Could you check a few things on this model? Use its own coordinates, in mm. Give positions to 0.01 mm unless a question says otherwise; leave off trailing zeros. Loops run counter-clockwise (first coordinate to the right, second up) from the corner with the lowest first, then second, coordinate; pieces in that order, holes last. Notation, with made-up numbers: (32.5, -14) - (85.5, -14) arc R30 cw to (85.5, 20) - close; hole circle Ø7 at (6.5, 25). An arc over 180 degrees is marked (long way). One line per item, written item: value. Start each with the question number.
Q1. I want a section at C-C (z = -207). Please give me the cut outline in (x, y) (3 decimals), then the cut area to 3 significant figures.
Q2. I'm going to push flat-ended pins straight in: P1, Ø2.5, axis at x = 189.47, z = -178, coming from the +Y side; P2, Ø1, axis at y = 2, z = -172, coming from the +X side. Where does each tip first touch, or does it pass through?
Q3. I want a section at B-B (x = 150). Please give me the cut outline in (y, z) (3 decimals).
Q4. I want a section at A-A (y = 2). Please give me the cut outline in (x, z).
Q5. If I drill on line 1 (Z direction, x = 189.5, y = 0.6); line 2 (Z direction, x = 271.5, y = 2.3); line 3 (Z direction, x = 96.5, y = 0.3), over which ranges is the centre line in solid material (lowest first)? Write a range as from..to.
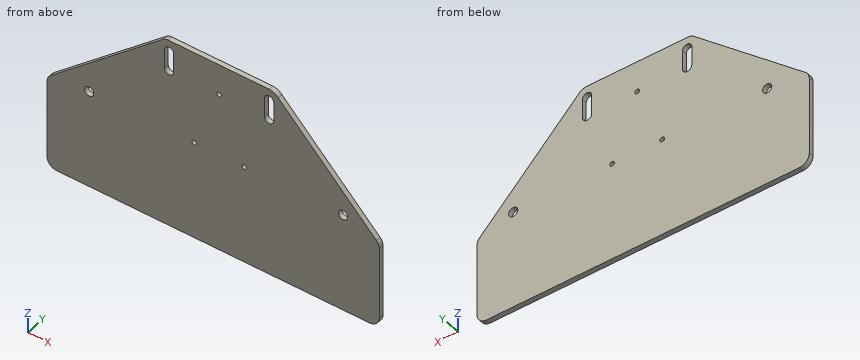
Autodesk Inventor part; units mm, degrees
ref_plane "YZ Plane" through (0, 0, 0) normal (1, 0, 0) x (0, 1, 0)
ref_plane "XZ Plane" through (0, 0, 0) normal (0, 1, 0) x (-1, 0, 0)
ref_plane "XY Plane" through (0, 0, 0) normal (0, 0, 1) x (1, 0, 0)
sketch "Sketch1" plane through (0, 0, 0) normal (0, 1, 0) x (-1, 0, 0)
  line L0 (-77.6185, -139.5068) -> (-293.5185, -139.5068)
  line L1 (-293.5185, -139.5068) -> (-293.5185, -291.9068)
  line L2 (-293.5185, -291.9068) -> (-77.6185, -291.9068)
  line L3 (-77.6185, -291.9068) -> (-77.6185, -139.5068)
  point P0 (0, 0)
  dimension "d0" = 215.9
  dimension "d1" = 152.4
extrude "Extrusion1" add sketch "Sketch1" along normal blind 3.175
sketch "Sketch2" plane through (0, 3.175, 0) normal (0, 1, 0) x (1, 0, 0)
  line L0 (77.6185, 291.9068) -> (77.6185, 139.5068)
  line L1 (77.6185, 139.5068) -> (293.5185, 139.5068)
  line L2 (293.5185, 139.5068) -> (293.5185, 291.9068)
  line L3 (293.5185, 291.9068) -> (77.6185, 291.9068)
  point P0 (0, 0)
  point P1 (156.9685, 165.5068)
  point P2 (104.9685, 218.5068)
  point P3 (269.9685, 218.5068)
  point P4 (221.9685, 165.5068)
  dimension "d4" = 144.35
  dimension "d5" = 26
  dimension "d7" = 79
  dimension "d19" = 27.35
  dimension "d20" = 79
  dimension "d21" = 26
  dimension "d22" = 79.35
  dimension "d23" = 192.35
hole "Hole1" at (156.9685, 3.175, -165.5068) at (104.9685, 3.175, -218.5068) at (269.9685, 3.175, -218.5068) at (221.9685, 3.175, -165.5068) direction (0, -1, 0) diameter 6 end through all
sketch "Sketch3" plane through (0, 3.175, 0) normal (0, 1, 0) x (1, 0, 0)
  line L0 (155.9994, 158.0068) -> (221.9685, 158.0068)
  circle A0 centre (221.9685, 165.5068) radius 3
  circle A1 centre (104.3905, 218.5068) radius 3
  circle A2 centre (156.9685, 165.5068) radius 3
  line L1 (153.2717, 158.9097) -> (79.8868, 220.4869)
  line L2 (77.6185, 139.5068) -> (293.5185, 139.5068)
  line L3 (293.5185, 229.1509) -> (293.5185, 276.0791)
  line L4 (293.5185, 291.9068) -> (77.6185, 291.9068)
  line L5 (77.6185, 291.9068) -> (77.6185, 139.5068)
  arc A3 (153.2717, 158.9097) -> (155.9994, 158.0068) centre (156.9685, 165.5068) ccw
  line L6 (96.6333, 206.4349) -> (77.6185, 222.3902)
  line L7 (48.2791, 233.5068) -> (391.5458, 233.5068) construction
  arc A4 (221.9685, 158.0068) -> (227.8466, 160.8487) centre (221.9685, 165.5068) ccw
  line L8 (227.8466, 160.8487) -> (291.6586, 224.6608)
  line L9 (293.5185, 226.5206) -> (293.5185, 282.4291)
  line L10 (293.5185, 139.5068) -> (293.5185, 291.9068)
  line L11 (287.1685, 282.4291) -> (83.9685, 282.4291)
  line L12 (77.6185, 276.0791) -> (77.6185, 225.3513)
  line L13 (77.6185, 291.9068) -> (77.6185, 139.5068)
  arc A5 (293.5185, 276.0791) -> (287.1685, 282.4291) centre (287.1685, 276.0791) ccw
  arc A6 (83.9685, 282.4291) -> (77.6185, 276.0791) centre (83.9685, 276.0791) ccw
  arc A7 (77.6185, 225.3513) -> (79.8868, 220.4869) centre (83.9685, 225.3513) ccw
  arc A8 (291.6586, 224.6608) -> (293.5185, 229.1509) centre (287.1685, 229.1509) ccw
  point P0 (0, 0)
  point P1 (77.6185, 282.4291)
  point P2 (77.6185, 160.8487)
  dimension "d24" = 7.5
  dimension "d40" = 98.7582
  dimension "d72" = 6
  dimension "d93" = 7.5
  dimension "d96" = 52.578
  dimension "d99" = 135
  dimension "d100" = 6.35
  dimension "d101" = 6.35
  dimension "d102" = 6.35
  dimension "d103" = 6.35
  dimension "d104" = 140
extrude "Extrusion3" cut sketch "Sketch3" against normal blind 25.4 contours L0 A4 L8 A8 L9 L10 L2 L5 L6 L1 A3 | L6 L5 A7 | A5 L11 A6 L5 L4 L10 L9
sketch "Sketch7" plane through (0, 3.175, 0) normal (0, 1, 0) x (1, 0, 0)
  circle A0 centre (156.9685, 165.5068) radius 3
  line L0 (155.9994, 158.0068) -> (221.9685, 158.0068)
  circle A1 centre (156.9685, 178.0036) radius 2.9972
  line L1 (153.9713, 178.0036) -> (153.9713, 165.3773)
  line L2 (159.9657, 178.0043) -> (159.9685, 165.5075)
  circle A2 centre (221.9713, 178.0036) radius 2.9972
  circle A3 centre (221.9685, 165.5068) radius 3
  line L3 (218.9741, 178.016) -> (218.9741, 165.3232)
  line L4 (224.9685, 178.0036) -> (224.9685, 165.5068)
  point P0 (0, 0)
  point P1 (218.9685, 165.5082)
  dimension "d76" = 5.9944
  dimension "d77" = 12.4968
  dimension "d78" = 5.9944
  dimension "d79" = 12.4968
  dimension "d88" = 6
extrude "Extrusion4" cut sketch "Sketch7" against normal blind 25.4 contours A0 L1 A1 L2 | A1
sketch "Sketch8" plane through (0, 3.175, 0) normal (0, 1, 0) x (1, 0, 0)
  arc A0 (224.9685, 178.0036) -> (218.9741, 177.9913) centre (221.9713, 178.0036) ccw
  circle A1 centre (221.9685, 165.5068) radius 3
  line L0 (218.9741, 178.016) -> (218.9741, 165.3232)
  line L1 (224.9685, 178.0036) -> (224.9685, 165.5068)
  point P0 (0, 0)
  point P1 (218.9685, 165.5082)
  dimension "d82" = 5.9944
  dimension "d83" = 12.4968
extrude "Extrusion5" cut sketch "Sketch8" against normal blind 25.4 contours L1 A1 L0 A0 | A1 L0 picked at (221.9464, 164.5591)
sketch "Sketch9" plane through (0, 3.175, 0) normal (0, 1, 0) x (1, 0, 0)
  point P0 (0, 0)
sketch "Sketch5" plane through (0, 3.175, 0) normal (0, 1, 0) x (1, 0, 0)
  circle A0 centre (104.9685, 218.5068) radius 3
  circle A1 centre (104.9685, 218.5068) radius 22.225
  circle A2 centre (156.9685, 165.5068) radius 3
  circle A3 centre (156.9685, 165.5068) radius 22.225
  circle A4 centre (221.9685, 165.5068) radius 3
  circle A5 centre (221.9685, 165.5068) radius 22.225
  circle A6 centre (269.9685, 218.5068) radius 3
  circle A7 centre (269.9685, 218.5068) radius 22.225
  line L0 (155.9994, 158.0068) -> (221.9685, 158.0068)
  line L1 (274.8943, 278.8204) -> (98.1742, 278.8204)
  arc A8 (224.9685, 178.0036) -> (218.9741, 178.016) centre (221.9713, 178.0036) ccw
  point P0 (0, 0)
  point P1 (205.7185, 218.5096)
  point P2 (189.4685, 178.0036)
  point P3 (173.2185, 218.5096)
  dimension "d45" = 44.45
  dimension "d47" = 44.45
  dimension "d48" = 44.45
  dimension "d49" = 44.45
  dimension "d50" = 60.5028
  dimension "d52" = 65
  dimension "d53" = 16.25
  dimension "d54" = 16.25
  dimension "d55" = 60.5028
  dimension "d58" = 52
  dimension "d62" = 32.5
  dimension "d95" = 60.3136
  dimension "d125" = 0
hole "Hole2" at (205.7185, 3.175, -218.5096) at (189.4685, 3.175, -178.0036) at (173.2185, 3.175, -218.5096) direction (0, -1, 0) diameter 3 end through all
sketch "Sketch11" plane through (0, 3.175, 0) normal (0, 1, 0) x (1, 0, 0)
  circle A0 centre (18.0131, 10.4316) radius 1.3525
  circle A1 centre (18.0131, 10.4316) radius 1.3525
  circle A2 centre (18.0131, 24.2612) radius 1.3525
  circle A3 centre (18.0131, 24.2612) radius 1.3525
  circle A4 centre (31.8426, 24.2612) radius 1.3525
  circle A5 centre (31.8426, 24.2612) radius 1.3525
  circle A6 centre (31.8426, 10.4316) radius 1.3525
  circle A7 centre (31.8426, 10.4316) radius 1.3525
  circle A8 centre (104.9685, 218.5068) radius 3
  point P0 (0, 0)
  point P1 (24.9279, 17.3464)
  point P2 (24.9279, 17.3464)
  dimension "d126" = 13.8296
  dimension "d127" = 13.8296
  dimension "d128" = 6.9148
  dimension "d129" = 6.9148
equation "\"d78\" = d76"
equation "\"d79\" = d77"
equation "\"d82\" = d84"
equation "\"d83\" = d85"
equation "\"d47\" = d45"
equation "\"d48\" = d45"
equation "\"d49\" = d48"
properties part number "track side panel V1"
Worked answers:
1. outline: (95.96, 0) - (273.998, 0) - (273.998, 3.175) - (95.96, 3.175) - close
1. area: 565 mm²
2. P1: passes through
2. P2: stops at x = 239.5
3. outline: (0, -282.429) - (3.175, -282.429) - (3.175, -161.655) - (0, -161.655) - close
4. outline: (77.62, -276.08) arc R6.35 ccw to (83.97, -282.43) - (287.17, -282.43) arc R6.35 ccw to (293.52, -276.08) - (293.52, -229.15) arc R6.35 ccw to (291.66, -224.66) - (227.85, -160.85) arc R7.5 ccw to (221.97, -158.01) - (156, -158.01) arc R7.56 ccw to (153.27, -158.91) - (79.89, -220.49) arc R6.35 ccw to (77.62, -225.35) - close; hole circle Ø6 at (104.97, -218.51); hole (153.97, -178) arc R3 ccw to (159.97, -178) - (159.97, -165.51) arc R3 ccw to (153.97, -165.38) - close; hole circle Ø3 at (173.22, -218.51); hole circle Ø3 at (189.47, -178); hole circle Ø3 at (205.72, -218.51); hole (218.97, -177.99) arc R3 ccw to (224.97, -178) - (224.97, -165.51) arc R3 ccw (long way) to (218.97, -165.69) - close; hole circle Ø6 at (269.97, -218.51)
5. line 1: z = -282.43..-179.5, -176.5..-158.01
5. line 2: z = -282.43..-221.09, -215.93..-204.5
5. line 3: z = -282.43..-206.55
